The figure shows three views and two pictorial views of one solid part (mm, origin at its lowest corner). Answer the questions. A direction names the side the tool comes from. Round coordinates to 2 decimals unless told otherwise and drop trailing zeros. Order: outer loops, then holes, each group sorted by start corner. A loop starts at its lowest first (then second) coordinate and runs counter-clockwise, first axis right, second up. Notation, with made-up numbers: (87.25, 0.25) -> (124.25, 0.25) arc R20 ccw to (124.25, 36.25) -> close; hole circle Ø10 at (-7, 9.5). An arc over 180 degrees is marked (long way). One line per item, written item: value. Start each with the question number.
1. Flat-ended cylindrical pins translate along their axes: pin 1 Ø2 at (x, z) = (22.5, 10) entering from -Y; pin 2 Ø1 at (x, y) = (22.5, 3) entering from +Z; pin 3 Ø1.5 at (x, y) = (3, 15.5) entering from -Z; pin 4 Ø4 at (y, z) = (10, 10) entering from -X. Find the tip coordinate at first contact, or state that the pin passes through.
2. Section D-D (x = 8.75) is taken. Give the vertices of the cut face in (y, z).
3. Consider line 1 (Y direction, x = 21.5, z = 13); line 2 (Y direction, x = 22.5, z = 3.75); line 3 (Z direction, x = 3.5, y = 6.25). Determine where each line is inside the solid, lowest interval first.
4. For the marked faces 1 and 2, determine the directions among +Z, -Z, +X, -X, +Y, -Y from which every point of the face is accessible in a straight line to the end or side of a thin tool.
5. Section A-A (z = 10) is taken. Give the vertices of the cut face in (x, y), then the cut area to 3 significant figures.
6. The mould has two halves that part along Y. Classify the marked faces 3, 4 and 5: released by +Y, released by -Y, zero draft, split by the parting line, or undercut.
7. Section B-B (x = 22.5) is taken. Give the vertices of the cut face in (y, z), then the cut area to 3 significant figures.
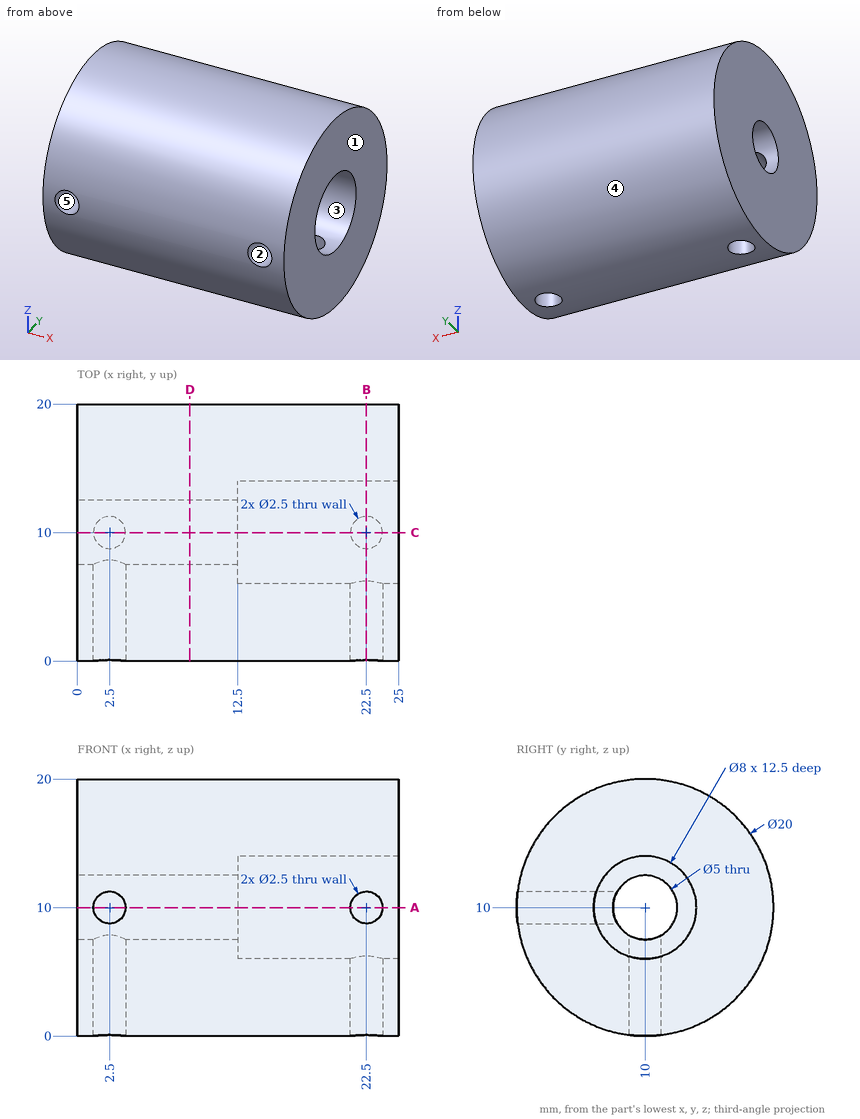
Answer:
1. pin 1: y = 13.87
1. pin 2: z = 17.6
1. pin 3: z = 1.2
1. pin 4: through
2. outline: circle Ø20 at (10, 10); hole circle Ø5 at (10, 10)
3. line 1: 0.46 to 7.35, 12.65 to 19.54
3. line 2: 2.19 to 8.75, 11.25 to 17.81
3. line 3: 0.73 to 9.25, 10.75 to 19.27
4. face 1: +Z, -Z, +X, +Y, -Y
4. face 2: -Y
5. outline: (0, 0) -> (1.25, 0) -> (1.25, 7.5) -> (0, 7.5) -> close; (0, 12.5) -> (12.5, 12.5) -> (12.5, 14) -> (25, 14) -> (25, 20) -> (0, 20) -> close; (3.75, 0) -> (21.25, 0) -> (21.25, 6) -> (12.5, 6) -> (12.5, 7.5) -> (3.75, 7.5) -> close; (23.75, 0) -> (25, 0) -> (25, 6) -> (23.75, 6) -> close
5. area: 304 mm^2
6. face 3: undercut
6. face 4: split by the parting line
6. face 5: zero draft
7. outline: (0.08, 8.75) arc R10 ccw to (8.75, 0.08) -> (8.75, 6.2) arc R4 cw to (6.2, 8.75) -> close; (0.08, 11.25) -> (6.2, 11.25) arc R4 cw (long way) to (11.25, 6.2) -> (11.25, 0.08) arc R10 ccw (long way) to start
7. area: 234 mm^2
